Build history of the part. All positions in model axes, mm. A direction names the side the tool comes from. Coordinates: 2 decimals unless noted, no trailing zeros. Write each loop counter-clockwise with the first axis right and the second up, starting at its lowest first coordinate (ties: lowest second). Pieces come first, ordered by that corner, then holes. Notation, with made-up numbers: (22.25, -9) -> (72.25, -9) arc R26 cw to (72.25, 28) -> close; hole circle Ø3 at (20, 11). An arc over 180 degrees is marked (long way). Write each question's results on one line, items separated by ' | '. Start each with the question number.
Q1. Drill centre lines: line 1 (Y direction, x = -62, z = 1.3); line 2 (Y direction, x = -75, z = 3.6); line 3 (Z direction, x = -84.5, y = 61.5). Where is each one in solid material? Low to high.
Q2. Two-plate mould, pull along Y, no slides. Class faces 6 (the face through (-71.842, 68, 2)), 7 (the face through (-63.534, 52.248, 2.687)), 8 (the face through (-75.099, 39.425, 4.943)): released by +Y, released by -Y, zero draft, split by the parting line, or undercut.
Q3. Tool access for faces 1 (the face through (-74.59, 64.32, 4.94)), 2 (the face through (-77.842, 68, 2)), 3 (the face through (-68.376, 49.191, 2.884)), 4 (the face through (-86, 44, 3.2)), 5 (the face through (-87.233, 41.172, 1.578)): list every direction of +Z, -Z, +X, -X, +Y, -Y with a clear straight run to the whole face (end or side of a thin tool).
Q4. Drop flat-ended pins along their axis: pin 1 Ø4 at (x, y) = (-61.53, 44.19) entering from -Z; pin 2 Ø1.6 at (y, z) = (68.5, 1.5) entering from -X; pin 3 Ø2 at (y, z) = (55.5, 4.5) entering from -X; pin 4 Ø2 at (x, y) = (-87.34, 51.87) entering from -Z. Give the stop position or say it passes through.
Q5. Saw through at C-C on y = 52.5. Count the separate pieces of the cut face and the enclosed holes in it, and give its area (3 significant figures).
Q6. Saw through at B-B on y = 43.5. Give the cut face in (x, z).
Q7. Saw through at A-A on z = 2.05. Give the cut face in (x, y).
from build123d import *

# Parameters (mm, degrees)
ESQUISSE1_R             = 17.97
BOSS_EXTRU_1_DEPTH      = 4.45
ESQUISSE2_R             = 12.45
BOSS_EXTRU_2_DEPTH      = 1
CHANFREIN1_SIZE         = 0.5
ESQUISSE5_R             = 1.5
ENL_V_MAT_EXTRU_1_DEPTH = 6.45
ESQUISSE6_R             = 3.5
ENL_V_MAT_EXTRU_2_DEPTH = 6.45
ESQUISSE7_R             = 7
ENL_V_MAT_EXTRU_3_DEPTH = 5
ENL_V_MAT_EXTRU_4_DEPTH = 3.2
CHANFREIN2_SIZE         = 0.2
ESQUISSE9_R             = 1.25
ENL_V_MAT_EXTRU_5_DEPTH = 6.45


with BuildPart() as part:
    # Esquisse1 → Boss.-Extru.1 (new body)
    with BuildSketch(Plane.XY):
        with Locations((-74.842203198, 51.872077922)):
            Circle(ESQUISSE1_R)
    extrude(amount=BOSS_EXTRU_1_DEPTH)

    # Esquisse2 → Boss.-Extru.2 (add)
    with BuildSketch(Plane.XY.offset(4.45)):
        with Locations((-74.842203198, 51.872077922)):
            Circle(ESQUISSE2_R)
    extrude(amount=BOSS_EXTRU_2_DEPTH)

    # Chanfrein1
    chanfrein1_edges = [part.edges().sort_by_distance(p)[0] for p in [
        (-92.812203198, 51.872077922, 0),
    ]]
    chamfer(chanfrein1_edges, length=CHANFREIN1_SIZE)

    # Esquisse5 → Enlèv. mat.-Extru.1 (cut, through all)
    with BuildSketch(Plane(origin=(0, 0, 0), x_dir=(-1, 0, 0), z_dir=(0, 0, -1))):
        with Locations((74.842203198, 67.242077922)):
            Circle(ESQUISSE5_R)
        with Locations((61.531392742, 44.187077922)):
            Circle(ESQUISSE5_R)
        with Locations((88.153013654, 44.187077922)):
            Circle(ESQUISSE5_R)
    extrude(amount=-ENL_V_MAT_EXTRU_1_DEPTH, mode=Mode.SUBTRACT)

    # Esquisse6 → Enlèv. mat.-Extru.2 (cut, through all)
    with BuildSketch(Plane(origin=(0, 0, 0), x_dir=(-1, 0, 0), z_dir=(0, 0, -1))):
        with Locations((74.842203198, 51.872077922)):
            Circle(ESQUISSE6_R)
    extrude(amount=-ENL_V_MAT_EXTRU_2_DEPTH, mode=Mode.SUBTRACT)

    # Esquisse7 → Enlèv. mat.-Extru.3 (cut)
    with BuildSketch(Plane.XY.offset(5.45)):
        with Locations((-74.842203198, 51.872077922)):
            Circle(ESQUISSE7_R)
    extrude(amount=-ENL_V_MAT_EXTRU_3_DEPTH, mode=Mode.SUBTRACT)

    # Esquisse8 → Enlèv. mat.-Extru.4 (cut)
    with BuildSketch(Plane(origin=(0, 0, 0), x_dir=(-1, 0, 0), z_dir=(0, 0, -1))):
        with BuildLine():
            Line((71.842203198, 70.411905134), (71.842203198, 66.363654544))
            ThreePointArc((71.842203198, 66.363654544), (74.842203198, 63.363654544), (77.842203198, 66.363654544))
            Line((77.842203198, 66.363654544), (77.842203198, 70.411905134))
            Line((77.842203198, 70.411905134), (71.842203198, 70.411905134))
        make_face()
        with BuildLine():
            Line((60.379554388, 39.925212907), (63.849582418, 42.010216097))
            ThreePointArc((63.849582418, 42.010216097), (64.875970095, 46.126832224), (60.759353968, 47.153219901))
            Line((60.759353968, 47.153219901), (57.289325938, 45.068216711))
            Line((57.289325938, 45.068216711), (60.379554388, 39.925212907))
        make_face()
        with BuildLine():
            Line((92.371338943, 45.133431645), (88.865451092, 47.15755694))
            ThreePointArc((88.865451092, 47.15755694), (84.76737488, 46.059480728), (85.865451092, 41.961404517))
            Line((85.865451092, 41.961404517), (89.371338943, 39.937279222))
            Line((89.371338943, 39.937279222), (92.371338943, 45.133431645))
        make_face()
    extrude(amount=-ENL_V_MAT_EXTRU_4_DEPTH, mode=Mode.SUBTRACT)

    # Chanfrein2
    chanfrein2_edges = [part.edges().sort_by_distance(p)[0] for p in [
        (-81.842203198, 51.872077922, 5.45),
    ]]
    chamfer(chanfrein2_edges, length=CHANFREIN2_SIZE)

    # Esquisse9 → Enlèv. mat.-Extru.5 (cut, through all)
    with BuildSketch(Plane(origin=(0, 0, 0), x_dir=(-1, 0, 0), z_dir=(0, 0, -1))):
        with Locations((62.342203198, 51.872077922)):
            Circle(ESQUISSE9_R)
        with Locations((87.342203198, 51.872077922)):
            Circle(ESQUISSE9_R)
    extrude(amount=-ENL_V_MAT_EXTRU_5_DEPTH, mode=Mode.SUBTRACT)


solid = part.part
Returned:
1) line 1: y = 39.3 to 40.9, 47.57 to 50.67, 53.07 to 64.44 | line 2: y = 33.9 to 44.87, 58.87 to 65.75, 68.73 to 69.84 | line 3: z = 0 to 4.45
2) face 6: zero draft | face 7: undercut | face 8: released by -Y
3) face 1: +Z, +Y | face 2: -Z, +Y | face 3: +Z | face 4: -Z | face 5: -Z, -X
4) pin 1: stops at z = 3.2 | pin 2: stops at x = -83.35 | pin 3: stops at x = -92.62 | pin 4: passes through
5) separate pieces: 4 | enclosed holes: 0 | area: 90.3 mm2
6) outline: (-90.74, 3.2) -> (-89.49, 3.2) -> (-89.49, 4.45) -> (-90.74, 4.45) -> close; (-86.82, 3.2) -> (-84.56, 3.2) -> (-84.56, 0) -> (-65.1, 0) -> (-65.1, 3.2) -> (-62.86, 3.2) -> (-62.86, 4.45) -> (-65.63, 4.45) -> (-65.63, 5.45) -> (-84.06, 5.45) -> (-84.06, 4.45) -> (-86.82, 4.45) -> close; (-60.2, 3.2) -> (-58.94, 3.2) -> (-58.94, 4.45) -> (-60.2, 4.45) -> close
7) outline: (-91.66, 45.54) -> (-88.87, 47.16) arc R3 cw to (-85.87, 41.96) -> (-88.64, 40.36) arc R17.97 ccw to (-61.06, 40.34) -> (-63.85, 42.01) arc R3 cw to (-60.76, 47.15) -> (-58.03, 45.52) arc R17.97 ccw to (-71.84, 69.59) -> (-71.84, 66.36) arc R3 cw to (-77.84, 66.36) -> (-77.84, 69.59) arc R17.97 ccw to start; hole circle Ø2.5 at (-87.34, 51.87); hole circle Ø14 at (-74.84, 51.87); hole circle Ø2.5 at (-62.34, 51.87)
